Verification items for the finished model (mm, model axes). Face numbers are marked on the shaded views. A direction names the side the tool comes from. Coordinates: 2 decimals unless noted, no trailing zeros. Order: outer loops, then holes, each group sorted by start corner. A loop starts at its lowest first (then second) coordinate and runs counter-clockwise, first axis right, second up. Notation, with made-up numbers: M 24.5,14 L 81.5,14 A27 cw 81.5,41 Z; hole C 15.5,50 d4. An arc over 180 degrees is marked long. Write item = value, one per line.
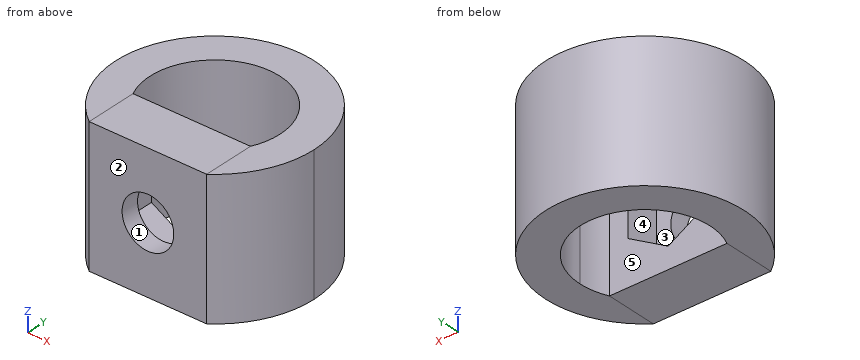
```python
from build123d import *

# Parameters (mm, degrees)
BOSS_EXTRU_1_DEPTH = 5.5
ESQUISSE5_W        = 19.1
ESQUISSE5_H        = 22.054780284
ESQUISSE5_R        = 4.2
BOSS_EXTRU_7_DEPTH = 3
BOSS_EXTRU_8_START = -11.02739
BOSS_EXTRU_8_DEPTH = 22.05478


with BuildPart() as part:
    # Esquisse1 → Boss.-Extru.1 (new body)
    with BuildSketch(Plane(origin=(0, 0, 0), x_dir=(1, 0, 0), z_dir=(0, 1, 0))):
        Polygon((-9.55, -5.513695071), (0, -11.027390142), (9.55, -5.513695071), (9.55, 5.513695071), (0, 11.027390142), (-9.55, 5.513695071), align=None)
        Polygon((0, -7.563288526), (6.55, -3.781644263), (6.55, 3.781644263), (0, 7.563288526), (-6.55, 3.781644263), (-6.55, -3.781644263), align=None, mode=Mode.SUBTRACT)
        Polygon((-9.55, -11.027390142), (0, -11.027390142), (-9.55, -5.513695071), align=None)
        Polygon((-9.55, 5.513695071), (0, 11.027390142), (-9.55, 11.027390142), align=None)
        Polygon((0, 11.027390142), (9.55, 5.513695071), (9.55, 11.027390142), align=None)
        Polygon((9.55, -11.027390142), (9.55, -5.513695071), (0, -11.027390142), align=None)
    extrude(amount=BOSS_EXTRU_1_DEPTH)

    # Esquisse5 → Boss.-Extru.7 (add)
    with BuildSketch(Plane(origin=(0, 0, 0), x_dir=(-1, 0, 0), z_dir=(0, -1, 0))):
        Rectangle(ESQUISSE5_W, ESQUISSE5_H)
        Circle(ESQUISSE5_R, mode=Mode.SUBTRACT)
    extrude(amount=BOSS_EXTRU_7_DEPTH)

    # Esquisse6 → Boss.-Extru.8 (add)
    with BuildSketch(Plane.XY.offset(BOSS_EXTRU_8_START)):
        with BuildLine():
            ThreePointArc((16.130793533, 10), (-7.285376509, 24.39186538), (-9.55, -3))
            Line((-9.55, -3), (-9.55, 5.5))
            ThreePointArc((-9.55, 5.5), (-2.305659544, 20.302253834), (10.557106611, 10))
            ThreePointArc((10.557106611, 10), (10.302253834, 7.694340456), (9.55, 5.5))
            Line((9.55, 5.5), (9.55, -3))
            ThreePointArc((9.55, -3), (14.39186538, 2.714623491), (16.130793533, 10))
        make_face()
    extrude(amount=BOSS_EXTRU_8_DEPTH)


solid = part.part
```
Item 1: Sectioned sample at B-B, the plane z = -9.25. Enter the section's corners in (x, y), then the cut area to 3 significant figures.
Report:
outline = M -9.55,-3 L 9.55,-3 A16.13 ccw long Z; hole M -9.55,5.5 L 9.55,5.5 A10.56 ccw long Z
area = 510 mm^2
Item 2: Release check for a two-part mould opening along Y. For the marked faces 1, 2 and 3 record: pulls with the +Y half, pulls with the -Y half, needs draft (parallel to the pull), parting line crosses it, or undercut.
Report:
face_1 = needs draft
face_2 = pulls with the -Y half
face_3 = undercut
Item 3: Scan lines: L1, parallel to Y at x = 0, z = 5; L2, parallel to Z at x = 0, y = -0.7; L3, parallel to Y at x = 0, z = 8. Record each from-to range of solid material in increasing order. Write a range as from..to.
Report:
L1 = -3..0, 20.56..26.13
L2 = -11.03..-4.2, 4.2..11.03
L3 = -3..5.5, 20.56..26.13
Item 4: Tool access check on the marked faces 4 and 5. Record the directions out of +Z, -Z, +X, -X, +Y, -Y that give a thin tool (end or side, any length) a straight path to the whole face; none if there is none.
Report:
face_4 = none
face_5 = +Z, -Z
Item 5: Sectioned sample at A-A, the plane y = 11.5. Enter the section's corners in (x, z).
Report:
outline = M -16.06,-11.03 L -10.45,-11.03 L -10.45,11.03 L -16.06,11.03 Z; M 10.45,-11.03 L 16.06,-11.03 L 16.06,11.03 L 10.45,11.03 Z
Item 6: Sectioned sample at D-D, the plane y = 1.5. Enter the section's corners in (x, z), then the cut area to 3 significant figures.
Report:
outline = M -13.71,-11.03 L 13.71,-11.03 L 13.71,11.03 L -13.71,11.03 Z; hole M -6.55,-3.78 L 0,-7.56 L 6.55,-3.78 L 6.55,3.78 L 0,7.56 L -6.55,3.78 Z
area = 456 mm^2
Item 7: Gauge pin test, flat ends, axial feed: pin 1 (1 mm diameter, centred on y = 0, z = -2.5, fed in from +X); pin 2 (4.5 mm diameter, centred on y = 4, z = -1, fed in from -X); pin 3 (6 mm diameter, centred on y = 3, z = -1.5, fed in from +X); pin 4 (4 mm diameter, centred on x = 1.5, y = 8.5, fed in from +Z). Record the tip position at first contact, or that the pin passes through.
Report:
pin_1 = 13.04
pin_2 = -15.69
pin_3 = 15.63
pin_4 = through
Item 8: Sectioned sample at C-C, the plane x = -0.5. Enter the section's corners in (y, z), then the cut area to 3 significant figures.
Report:
outline = M -3,-11.03 L 5.5,-11.03 L 5.5,-7.27 L 0,-7.27 L 0,-4.17 L -3,-4.17 Z; M -3,4.17 L 0,4.17 L 0,7.27 L 5.5,7.27 L 5.5,11.03 L -3,11.03 Z; M 20.55,-11.03 L 26.12,-11.03 L 26.12,11.03 L 20.55,11.03 Z
area = 205 mm^2
